Could you check a few things on this model? Use its own coordinates, in mm. A direction names the side the tool comes from. Give positions to 0.01 mm unless a question says otherwise; leave off trailing zeros. Write each loop counter-clockwise with the first axis right and the second up, starting at its lowest first coordinate (ties: lowest second). Pieces come first, ordered by that corner, then holes. Notation, with made-up numbers: (24.25, 85) - (30.25, 85) arc R26 ccw to (30.25, 124) - close; hole circle Ø9 at (-10, -31.75). An arc over 180 degrees is marked (long way). Use one line per item in the form item = value.
```python
from build123d import *

# Parameters (mm, degrees)
ESQUISSE1_R                  = 3.5
BOSS_EXTRU_1_DEPTH           = 5
ESQUISSE4_R                  = 5.5
BOSS_EXTRU_3_DEPTH           = 1
ESQUISSE5_R                  = 10
BOSS_EXTRU_4_DEPTH           = 1
ESQUISSE6_R                  = 0.5
BOSS_EXTRU_5_DEPTH           = 4
BOSS_EXTRU_6_DEPTH           = 0.8
R_P_TITION_CIRCULAIRE1_COUNT = 3


with BuildPart() as part:
    # Esquisse1 → Boss.-Extru.1 (new body)
    with BuildSketch(Plane(origin=(0, 0, 0), x_dir=(1, 0, 0), z_dir=(0, 1, 0))):
        with Locations(Location((0, 0, 0), (0, 0, 270))):
            Circle(ESQUISSE1_R)
    extrude(amount=BOSS_EXTRU_1_DEPTH)

    # Esquisse4 → Boss.-Extru.3 (add)
    with BuildSketch(Plane(origin=(0, 5, 0), x_dir=(1, 0, 0), z_dir=(0, 1, 0))):
        with Locations(Location((0, 0, 0), (0, 0, 270))):
            Circle(ESQUISSE4_R)
    extrude(amount=BOSS_EXTRU_3_DEPTH)

    # Esquisse5 → Boss.-Extru.4 (add)
    with BuildSketch(Plane(origin=(0, 6, 0), x_dir=(1, 0, 0), z_dir=(0, 1, 0))):
        with Locations(Location((0, 0, 0), (0, 0, 270))):
            Circle(ESQUISSE5_R)
    extrude(amount=BOSS_EXTRU_4_DEPTH)

    # Esquisse6 → Boss.-Extru.5 (add)
    with BuildSketch(Plane(origin=(0, 7, 0), x_dir=(1, 0, 0), z_dir=(0, 1, 0))):
        with Locations(Location((0, 0, 0), (0, 0, 270))):
            Circle(ESQUISSE6_R)
    extrude(amount=BOSS_EXTRU_5_DEPTH)

    # Esquisse7 → Boss.-Extru.6 (add)
    with BuildSketch(Plane(origin=(0, 7, 0), x_dir=(1, 0, 0), z_dir=(0, 1, 0))):
        Polygon((0, 5), (0.5, 5), (0.5, 8), (-0.5, 8), (-0.5, 5), align=None)
    boss_extru_6 = extrude(amount=BOSS_EXTRU_6_DEPTH)

    # Répétition circulaire1: Boss.-Extru.6 ×3 about axis
    r_p_tition_circulaire1_axis = Axis((0, 0, 0), (0, 1, 0))
    for i in range(1, R_P_TITION_CIRCULAIRE1_COUNT):
        add(boss_extru_6.rotate(r_p_tition_circulaire1_axis, i * 360 / R_P_TITION_CIRCULAIRE1_COUNT))


solid = part.part
```
1. Imagine slicing it at A-A, the plane z = 0. List the corners of the cut face in (x, y) for me, and give its area (3 significant figures).
Response values:
outline = (-10, 6) - (-5.5, 6) - (-5.5, 5) - (-3.5, 5) - (-3.5, 0) - (3.5, 0) - (3.5, 5) - (5.5, 5) - (5.5, 6) - (10, 6) - (10, 7) - (0.5, 7) - (0.5, 11) - (-0.5, 11) - (-0.5, 7) - (-10, 7) - close
area = 70.0 mm²
2. If we mould it in two halves opening along X, with no side actions, what happens to faces 6 (the face through (-4, 6, 4)), 7 (the face through (-5.397, 7.394, 3.694)), 8 (the face through (5.36, 7.39, 3.67)), 9 (the face through (-5.861, 7.394, 2.806))? For each: pulls with the +X half, pulls with the -X half, needs draft (parallel to the pull), parting line crosses it, or undercut.
Response values:
face_6 = needs draft
face_7 = undercut
face_8 = undercut
face_9 = pulls with the -X half
3. Imagine slicing it at C-C, the plane y = 10. List the corners of the cut face in (x, z) for me.
Response values:
outline = circle Ø1 at (0, 0)
4. For pin 1 (5 mm diameter, centred on x = -4.5, y = 6.5, fed in from +Z); pin 2 (2 mm diameter, centred on y = 2.5, z = 0.5, fed in from +X); pin 3 (0.9 mm diameter, centred on y = 7.5, z = -7, fed in from -X), each with a flat end and sliding along its axis, tell me the tip position at first contact or that it passes through.
Response values:
pin_1 = 9.8
pin_2 = 3.5
pin_3 = -0.5
5. If I drill on line 1 (Y direction, x = 8, z = -5); line 2 (Y direction, x = -3, z = -4.5); line 3 (Z direction, x = 1, y = 4.5), over which ranges is the centre line in solid material (lowest first)? Write a range as from..to.
Response values:
line_1 = 6..7
line_2 = 5..7
line_3 = -3.35..3.35
6. Imagine slicing it at D-D, the plane z = -2.75. List the corners of the cut face in (x, y) for me, and give its area (3 significant figures).
Response values:
outline = (-9.61, 6) - (-4.76, 6) - (-4.76, 5) - (-2.17, 5) - (-2.17, 0) - (2.17, 0) - (2.17, 5) - (4.76, 5) - (4.76, 6) - (9.61, 6) - (9.61, 7) - (-9.61, 7) - close
area = 50.4 mm²
7. Imagine slicing it at B-B, the plane x = 3. List the corners of the cut face in (y, z) for me, and give its area (3 significant figures).
Response values:
outline = (0, -1.8) - (5, -1.8) - (5, -4.61) - (6, -4.61) - (6, -9.54) - (7, -9.54) - (7, 9.54) - (6, 9.54) - (6, 4.61) - (5, 4.61) - (5, 1.8) - (0, 1.8) - close
area = 46.3 mm²
8. Which directions (+Z, -Z, +X, -X, +Y, -Y) give clear straight access to the entire face, cutting with the end or side of a thin tool? Please do faces 1 (the face through (-5.6, 7.8, 3.3)), 2 (the face through (-0.488, 8.972, -0.108)), 3 (the face through (-5.37, 5.49, -1.19)), 4 (the face through (5.9, 7.39, 2.83)), 5 (the face through (0, 7.8, -7)).
Response values:
face_1 = +Z, -Z, +X, -X, +Y
face_2 = +Y
face_3 = -Y
face_4 = -Z, +X, +Y
face_5 = -Z, +X, -X, +Y
